Geometry check sheet. Reference: the model listing, model coordinates, mm. A direction names the side the tool comes from. Give positions to 0.01 mm unless a question says otherwise; leave off trailing zeros. Order: outer loops, then holes, each group sorted by start corner. A loop starts at its lowest first (then second) coordinate and runs counter-clockwise, first axis right, second up. Notation, with made-up numbers: M 56,-7 L 70,-7 A19 cw 70,26 Z; hole C 40,-12.5 d3. An arc over 180 degrees is marked long. Answer as CSV lines item,"result".
from build123d import *

# Parameters (mm, degrees)
F1_DEPTH       = 63.5
F0_W           = 25.4
F0_H           = 19.05
F2_DEPTH       = 25.4
F3_DEPTH       = 7.9375
F5_R           = 6.35
F7_D           = 13.49248
F7_CSINK_D     = 23.8252
F7_CSINK_ANGLE = 82


with BuildPart() as f1:
    # F0 (on Front) → F1 (new body, symmetric)
    with BuildSketch(Plane.XZ):
        Polygon((-41.275, 9.525), (-41.275, -9.525), (41.275, -9.525), (41.275, 9.525), (22.225, 9.525), align=None)
    extrude(amount=F1_DEPTH, both=True)

    # F0 (on Front) → F2 (join, symmetric)
    with BuildSketch(Plane.XZ):
        with BuildLine():
            Line((22.225, 9.525), (41.275, 9.525))
            Line((41.275, 9.525), (41.275, 27.0002))
            ThreePointArc((41.275, 27.0002), (45.9246798487, 38.2255201513), (57.15, 42.8752))
            Line((57.15, 42.8752), (60.325, 42.8752))
            Line((60.325, 42.8752), (60.325, 61.9252))
            Line((60.325, 61.9252), (57.15, 61.9252))
            add(Edge.make_bspline(
                [(56.4151043372, 61.9174672666), (56.659972062, 61.9205386908), (56.9049388479, 61.9231167628), (57.15, 61.9252)],
                knots=[110.9697423525, 110.9697423525, 110.9697423525, 110.9697423525, 111.5045361635, 111.5045361635, 111.5045361635, 111.5045361635], degree=3))
            ThreePointArc((56.4151043372, 61.9174672666), (32.1958234355, 51.4346980916), (22.225, 27.0002))
            Line((22.225, 27.0002), (22.225, 9.525))
        make_face()
        with Locations((73.025, 52.4002)):
            Rectangle(F0_W, F0_H)
    extrude(amount=F2_DEPTH, both=True)

    # F0 (on Front) → F3 (join, symmetric)
    with BuildSketch(Plane.XZ):
        with BuildLine():
            add(Edge.make_bspline(
                [(-41.275, 9.525), (-40.9398250429, 39.4009187199), (5.6050392748, 61.2801465881), (56.4151043372, 61.9174672666)],
                knots=[0, 0, 0, 0, 110.9697423525, 110.9697423525, 110.9697423525, 110.9697423525], degree=3))
            Line((-41.275, 9.525), (22.225, 9.525))
            Line((22.225, 9.525), (22.225, 27.0002))
            ThreePointArc((22.225, 27.0002), (32.1958234355, 51.4346980916), (56.4151043372, 61.9174672666))
        make_face()
    extrude(amount=F3_DEPTH, both=True)

    # F0 (on Front) → F4 (revolve)
    with BuildSketch(Plane.XZ):
        Polygon((85.725, 66.6865812632), (85.725, 61.9252), (85.725, 42.8752), (85.725, 38.1115812632), (111.125, 38.1115812632), (111.125, 66.6865812632), align=None)
    revolve(axis=Axis((85.725, 0, 52.3990812632), (0, 0, 1)))

    # F5
    f5_edges = [f1.edges().sort_by_distance(p)[0] for p in [
        (-41.275, -63.5, 0),
        (41.275, -63.5, 0),
        (41.275, 63.5, 0),
        (-41.275, 63.5, 0),
    ]]
    fillet(f5_edges, radius=F5_R)

    # F7 (through all)
    with Locations(Plane.XY.offset(66.6865812632)):
        with Locations((85.725, 0)):
            CounterSinkHole(F7_D / 2, F7_CSINK_D / 2, counter_sink_angle=F7_CSINK_ANGLE)


solid = f1.part
(1) Tool access check on faces 5 (the face through (80, -5, 38.112)), 6 (the face through (60, 2, 42.875)), 7 (the face through (32.46, 16.55, 51.7)). Record the directions out of +Z, -Z, +X, -X, +Y, -Y that give a thin tool (end or side, any length) a straight path to the whole face; none if there is none.
The answers:
face 5,"-Z, +X, +Y, -Y"
face 6,"-Z"
face 7,"+Z, -X, +Y"
(2) Section check C-C on x = 68.5. Enter the section's corners in (y, z).
The answers:
outline,"M -25.4,42.88 L -18.67,42.88 L -18.67,38.11 L 18.67,38.11 L 18.67,42.88 L 25.4,42.88 L 25.4,61.93 L 18.67,61.93 L 18.67,66.69 L -18.67,66.69 L -18.67,61.93 L -25.4,61.93 Z"
(3) Section check B-B on y = 42. Enter the section's corners in (x, z) (3 decimals), then the cut area to 3 significant figures.
The answers:
outline,"M -41.275,-9.525 L 41.275,-9.525 L 41.275,9.525 L -41.275,9.525 Z"
area,"1,570 mm2"
(4) Material ranges on line 1 (X direction, y = -14.5, z = 23.5) (3 decimals); line 2 (Z direction, x = 15.5, y = 49) (3 decimals); line 3 (Y direction, x = 2.5, z = 46), recorded low to high.
The answers:
line 1,"x = 22.225 to 41.275"
line 2,"z = -9.525 to 9.525"
line 3,"y = -7.94 to 7.94"
(5) Draft check along Y on faces 1 (the face through (-39.464, 61.59, -0.133)), 2 (the face through (92.465, 0.297, 49.269)), 3 (the face through (41.275, -1, 4)), 4 (the face through (46, -25.4, 42)). Enter one of: +Y half, -Y half, draft (parallel to the pull), parting line (faces both ways), or undercut.
The answers:
face 1,"+Y half"
face 2,"undercut"
face 3,"draft"
face 4,"-Y half"
(6) Gauge pin test, flat ends, axial feed: P1, Ø5, axis at y = -20, z = 22, coming from the -X side (3 decimals); P2, Ø14.5, axis at x = 72.5, y = 12, coming from the -Z side; P3, Ø4, axis at y = 15.5, z = 37.5, coming from the -X side. Record the tip position at first contact, or that the pin passes through.
The answers:
P1,"stops at x = 22.225"
P2,"stops at z = 38.11"
P3,"stops at x = 23.28"
(7) Section check A-A on z = 7. Enter the section's corners in (x, y) (3 decimals).
The answers:
outline,"M -41.275,-57.15 A6.35 ccw -34.925,-63.5 L 34.925,-63.5 A6.35 ccw 41.275,-57.15 L 41.275,57.15 A6.35 ccw 34.925,63.5 L -34.925,63.5 A6.35 ccw -41.275,57.15 Z"
